```python
from build123d import *

# Parameters (mm, degrees)
SKETCH1_W           = 150
SKETCH1_H           = 150
BOSS_EXTRUDE1_DEPTH = 8
SKETCH4_W           = 150
SKETCH4_H           = 150
SKETCH4_W_2         = 143
SKETCH4_H_2         = 143
BOSS_EXTRUDE2_DEPTH = 42
EXTRUDE_THIN1_DEPTH = 6
SKETCH6_W           = 2
SKETCH6_H           = 2
CUT_EXTRUDE1_DEPTH  = 143


with BuildPart() as part:
    # Sketch1 → Boss-Extrude1 (new body)
    with BuildSketch(Plane.XY):
        Rectangle(SKETCH1_W, SKETCH1_H)
    extrude(amount=BOSS_EXTRUDE1_DEPTH)

    # Sketch4 → Boss-Extrude2 (add)
    with BuildSketch(Plane.XY.offset(8)):
        Rectangle(SKETCH4_W, SKETCH4_H)
        Rectangle(SKETCH4_W_2, SKETCH4_H_2, mode=Mode.SUBTRACT)
    extrude(amount=BOSS_EXTRUDE2_DEPTH)

    # Sketch5 → Extrude-Thin1 (add)
    with BuildSketch(Plane.XY.offset(50)):
        Polygon((71.5, 71.5), (71.5, -71.5), (-71.5, -71.5), (-71.5, 71.5), (-75, 71.5), (-75, -75), (75, -75), (75, 71.5), align=None)
    extrude(amount=EXTRUDE_THIN1_DEPTH)

    # Sketch6 → Cut-Extrude1 (cut)
    with BuildSketch(Plane(origin=(0, 71.5, 0), x_dir=(1, 0, 0), z_dir=(0, 1, 0))):
        with Locations((71.5, -53)):
            Rectangle(SKETCH6_W, SKETCH6_H)
    cut_extrude1 = extrude(amount=-CUT_EXTRUDE1_DEPTH, mode=Mode.SUBTRACT)

    # Mirror1: Cut-Extrude1 across plane
    add(cut_extrude1.mirror(Plane(origin=(0, 0, 0), x_dir=(0, 0, 1), z_dir=(1, 0, 0))), mode=Mode.SUBTRACT)


solid = part.part
```
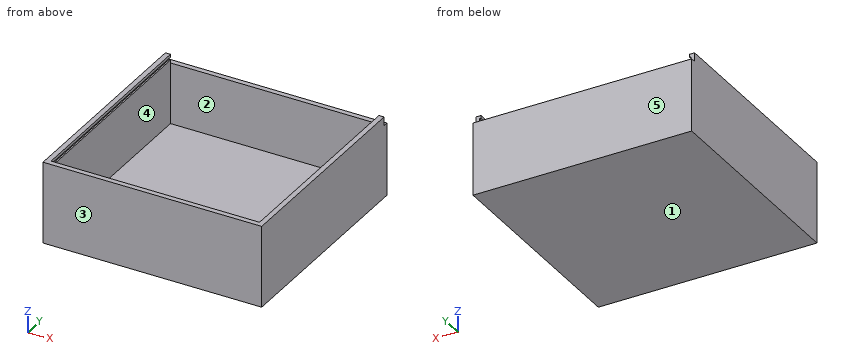
Design review of the part built by this model. Coordinates are the model's own, in mm. Face numbers are marked on the shaded views. A direction names the side the tool comes from. Coordinates: 2 decimals unless noted, no trailing zeros. Order: outer loops, then holes, each group sorted by start corner. A loop starts at its lowest first (then second) coordinate and runs counter-clockwise, first axis right, second up. Notation, with made-up numbers: (57.25, 12.25) - (76.25, 12.25) arc R23 ccw to (76.25, 27.25) - close; hole circle Ø4 at (61.25, 12.25). An arc over 180 degrees is marked (long way). Answer in a Markdown table with one row per item.
(1) Wall thickness on line 1 along X through (y, z) = (9, 21); line 2 along Y through (x, z) = (7.5, 53.5): over which ranges is each line inside the solid? List them lowest first. Write a range as from..to.
Checked values:
| item | result |
|---|---|
| line 1 | -75..-71.5, 71.5..75 |
| line 2 | -75..-71.5 |
(2) For the marked faces 4 and 5, list the 3-axis set-ups (+Z, -Z, +X, -X, +Y, -Y) from which the entire face can be reached by the end or side of a thin tool; tool diameter is ignored.
Checked values:
| item | result |
|---|---|
| face 4 | +Z |
| face 5 | +Z, -Z, +X, -X, +Y |
(3) Consider section B-B on y = -40.5. State the section outline as (x, z) points, plus the area to 3 significant figures.
Checked values:
| item | result |
|---|---|
| outline | (-75, 0) - (75, 0) - (75, 56) - (71.5, 56) - (71.5, 54) - (72.5, 54) - (72.5, 52) - (71.5, 52) - (71.5, 8) - (-71.5, 8) - (-71.5, 52) - (-72.5, 52) - (-72.5, 54) - (-71.5, 54) - (-71.5, 56) - (-75, 56) - close |
| area | 1,530 mm^2 |
(4) The part is to be moulded in two halves that separate along Y. For the marked faces 1, 2 and 3, say which applies: released by +Y, released by -Y, zero draft, split by the parting line, or undercut.
Checked values:
| item | result |
|---|---|
| face 1 | zero draft |
| face 2 | undercut |
| face 3 | released by -Y |
(5) Consider section C-C on x = -56. State the section outline as (y, z) points.
Checked values:
| item | result |
|---|---|
| outline | (-75, 0) - (75, 0) - (75, 50) - (71.5, 50) - (71.5, 8) - (-71.5, 8) - (-71.5, 56) - (-75, 56) - close |
(6) Clearance check with flat-ended pins moving along their axes: pin 1 (4 mm diameter, centred on x = 0.5, y = 73, fed in from +Z); pin 2 (4 mm diameter, centred on x = 20, y = -29.5, fed in from +Z); pin 3 (3 mm diameter, centred on x = 73.5, z = 52.5, fed in from +Y). State where each tip first meets the part, or that it passes through.
Checked values:
| item | result |
|---|---|
| pin 1 | z = 50 |
| pin 2 | z = 8 |
| pin 3 | y = 71.5 |
(7) Consider section A-A on z = 45. State the section outline as (x, y) points.
Checked values:
| item | result |
|---|---|
| outline | (-75, -75) - (75, -75) - (75, 75) - (-75, 75) - close; hole (-71.5, -71.5) - (71.5, -71.5) - (71.5, 71.5) - (-71.5, 71.5) - close |
